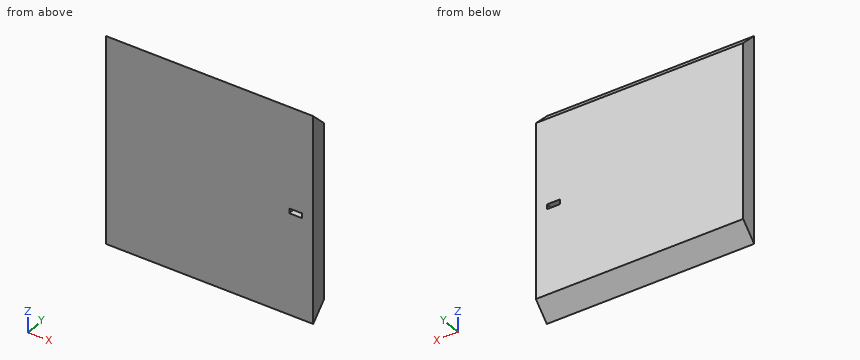
Autodesk Inventor part; units mm, degrees
ref_plane "YZ Plane" through (0, 0, 0) normal (1, 0, 0) x (0, 1, 0)
ref_plane "XZ Plane" through (0, 0, 0) normal (0, 1, 0) x (-1, 0, 0)
ref_plane "XY Plane" through (0, 0, 0) normal (0, 0, 1) x (1, 0, 0)
sketch "Sketch1" plane through (0, 0, 0) normal (0, 1, 0) x (-1, 0, 0)
  line L0 (-65, -65) -> (65, -65)
  line L1 (65, -65) -> (65, 65)
  line L2 (65, 65) -> (-65, 65)
  line L3 (-65, 65) -> (-65, -65)
  line L4 (-65, -65) -> (65, 65) construction
  line L5 (65, -65) -> (-65, 65) construction
  point P0 (0, 0)
  dimension "d0" = 130
  dimension "d1" = 130
extrude "Extrusion1" add sketch "Sketch1" along normal blind 10
chamfer "Chamfer1" distance 10 angle 45 2 edges at (0, 10, 65) (0, 10, -65)
sketch "Sketch2" plane through (0, 10, 0) normal (0, 1, 0) x (1, 0, 0)
  line L0 (58, -1.5) -> (50, -1.5)
  line L1 (50, -1.5) -> (50, 1.5)
  line L2 (50, 1.5) -> (58, 1.5)
  line L3 (58, 1.5) -> (58, -1.5)
  line L4 (58, -1.5) -> (50, 1.5) construction
  line L5 (50, -1.5) -> (58, 1.5) construction
  line L6 (65, -55) -> (65, 55)
  point P0 (0, 0)
  point P1 (54, 0)
  dimension "d7" = 8
  dimension "d8" = 3
  dimension "d9" = 7
extrude "Extrusion2" cut sketch "Sketch2" against normal blind 10
properties part number "inner_side"
Model file for the job. Use its own axes, mm. Coordinates: 2 decimals unless noted, no trailing zeros. Order: outer loops, then holes, each group sorted by start corner. A loop starts at its lowest first (then second) coordinate and runs counter-clockwise, first axis right, second up. Notation, with made-up numbers: (52, 3.5) - (89, 3.5) arc R13 cw to (89, 15.5) - close; hole circle Ø9 at (-35.5, 43). An arc over 180 degrees is marked (long way). Return JSON: item names as keys, results as strings. Group by question number.
1) Probe line 1 (Z direction, x = 7.5, y = 2); line 2 (Z direction, x = 52.5, y = 9.25); line 3 (Z direction, x = 32.5, y = 1.5). List the from-to ranges inside material, lowest first. Write a range as from..to.
2) Saw through at A-A, the plane y = 6. Write the cut outline in (x, z), plus the area to 3 significant figures.
3) Flat gauge pins, fed straight in: P1, Ø1.5, axis at x = -45.5, y = 9, coming from the +Z side; P2, Ø2, axis at x = -45.5, y = 2.5, coming from the -Z side; P3, Ø4, axis at x = 52, y = 5.5, coming from the -Z side. Where does each tip first touch, or does it go through?
Values found:
{
 "1": {"line 1": "z = -63..63", "line 2": "z = -55.75..-1.5, 1.5..55.75", "line 3": "z = -63.5..63.5"},
 "2": {"outline": "(-65, -59) - (65, -59) - (65, 59) - (-65, 59) - close; hole (50, -1.5) - (58, -1.5) - (58, 1.5) - (50, 1.5) - close", "area": "15,300 mm²"},
 "3": {"P1": "stops at z = 56.75", "P2": "stops at z = -63.5", "P3": "stops at z = -61.5"}
}
